The model under review builds one solid part; all positions refer to its coordinate system, in mm. A direction names the side the tool comes from. Coordinates: 2 decimals unless noted, no trailing zeros. Loops run counter-clockwise (first coordinate to the right, second up) from the corner with the lowest first, then second, coordinate; pieces in that order, holes last. Notation, with made-up numbers: M 74.5,-39.75 L 83.5,-39.75 A16 ccw 83.5,-30.75 Z; hole C -17,23.5 d10. An arc over 180 degrees is marked long. Return JSON: item names as keys, results as strings.
Autodesk Fusion 360 part; units mm, degrees
sketch "Sketch1" plane through (0, 0, 0) normal (0, 0, 1) x (1, 0, 0)
  line L0 (5, 5) -> (130, 5)
  line L1 (130, 5) -> (130, 205)
  line L2 (130, 205) -> (5, 205)
  line L3 (5, 205) -> (5, 5)
  line L4 (5, 5) -> (31.5, 5)
  line L5 (31.5, 5) -> (31.5, 45)
  line L6 (31.5, 45) -> (103.5, 45)
  line L7 (103.5, 45) -> (103.5, 184)
  line L8 (103.5, 184) -> (31.5, 184)
  line L9 (31.5, 184) -> (31.5, 45)
  line L10 (31.5, 45) -> (36.5, 45)
  line L11 (36.5, 45) -> (36.5, 50)
  circle A0 centre (36.5, 50) radius 1.75
  line L12 (103.5, 45) -> (98.5, 45)
  line L13 (98.5, 45) -> (98.5, 50)
  circle A1 centre (98.5, 50) radius 1.75
  line L14 (31.5, 184) -> (36.5, 184)
  line L15 (36.5, 184) -> (36.5, 179)
  circle A2 centre (36.5, 179) radius 1.75
  line L16 (103.5, 184) -> (103.5, 179)
  line L17 (103.5, 179) -> (98.5, 179)
  circle A3 centre (98.5, 179) radius 1.75
  dimension "d1" = 125
  dimension "d2" = 200
  dimension "d58" = 26.5
  dimension "d59" = 40
  dimension "d60" = 72
  dimension "d61" = 139
  dimension "d62" = 5
  dimension "d63" = 5
  dimension "d64" = 3.5
  dimension "d65" = 5
  dimension "d66" = 5
  dimension "d67" = 3.5
  dimension "d68" = 5
  dimension "d69" = 5
  dimension "d70" = 3.5
  dimension "d71" = 5
  dimension "d72" = 5
  dimension "d73" = 3.5
extrude "Extrude1" add sketch "Sketch1" along normal blind 3 contours L6 L7 L8 L9 L10 L12 L14 L16 | L0 L1 L2 L3 L4
sketch "Sketch2" plane through (0, 0, 0) normal (0, 0, -1) x (-1, 0, 0)
  line L0 (-5, 5) -> (-5, 205)
  line L1 (-5, 205) -> (-130, 205)
  line L2 (-130, 205) -> (-130, 5)
  line L3 (-130, 5) -> (-5, 5)
  line L4 (-130, 205) -> (-130, 185)
  line L5 (-130, 5) -> (-130, 25)
  line L6 (-130, 185) -> (-127, 185)
  line L7 (-127, 185) -> (-127, 25)
  line L8 (-127, 25) -> (-130, 25)
  line L9 (-130, 25) -> (-130, 185)
  line L10 (-8, 185) -> (-8, 25)
  line L11 (-5, 25) -> (-5, 185)
  line L12 (-5, 185) -> (-8, 185)
  line L13 (-5, 205) -> (-5, 185)
  line L14 (-8, 25) -> (-5, 25)
  line L15 (-5, 5) -> (-5, 25)
  line L16 (-5, 205) -> (-10.3033, 199.6967)
  line L17 (-5, 205) -> (-10, 205) construction
  line L18 (-5, 5) -> (-10.3033, 10.3033)
  line L19 (-5, 5) -> (-10, 5) construction
  circle A0 centre (-10.3033, 10.3033) radius 2.5
  circle A1 centre (-10.3033, 199.6967) radius 2.5
  circle A2 centre (-124.6967, 199.6967) radius 2.5
  line L20 (-130, 205) -> (-124.6967, 199.6967)
  line L21 (-130, 5) -> (-124.6967, 10.3033)
  circle A3 centre (-124.6967, 10.3033) radius 2.5
  line L22 (-67.5, 205) -> (-130, 205)
  line L23 (-67.5, 205) -> (-5, 205)
  line L24 (-30, 205) -> (-30, 5)
  line L25 (-30, 205) -> (-5, 205)
  line L26 (-5, 185) -> (-5, 205)
  line L27 (-5, 185) -> (-8, 185)
  line L28 (-8, 185) -> (-8, 25)
  line L29 (-8, 25) -> (-5, 25)
  line L30 (-5, 25) -> (-5, 5)
  line L31 (-5, 5) -> (-30, 5)
  line L32 (-30, 205) -> (-67.5, 205)
  line L33 (-67.5, 5) -> (-36.25, 5)
  line L34 (-67.5, 5) -> (-98.75, 5)
  line L35 (-67.5, 205) -> (-130, 205)
  line L36 (-130, 205) -> (-130, 185)
  line L37 (-127, 185) -> (-127, 25)
  line L38 (-130, 5) -> (-130, 25)
  line L39 (-130, 5) -> (-98.75, 5)
  line L40 (-130, 185) -> (-127, 185)
  line L41 (-30, 205) -> (-55, 205)
  line L42 (-55, 205) -> (-55, 5)
  line L43 (-55, 5) -> (-30, 5)
  line L44 (-30, 5) -> (-30, 205)
  line L45 (-55, 205) -> (-80, 205)
  line L46 (-80, 205) -> (-80, 5)
  line L47 (-80, 5) -> (-55, 5)
  line L48 (-55, 5) -> (-55, 205)
  line L49 (-80, 205) -> (-105, 205)
  line L50 (-105, 205) -> (-105, 5)
  line L51 (-105, 5) -> (-80, 5)
  line L52 (-80, 5) -> (-80, 205)
  circle A4 centre (-98.5, 50) radius 1.75
  circle A5 centre (-98.5, 179) radius 1.75
  circle A6 centre (-36.5, 50) radius 1.75
  circle A7 centre (-36.5, 179) radius 1.75
  dimension "d6" = 20
  dimension "d7" = 3
  dimension "d8" = 45
  dimension "d9" = 7.5
  dimension "d10" = 45
  dimension "d11" = 7.5
  dimension "d12" = 5
  dimension "d13" = 5
  dimension "d20" = 160
  dimension "d21" = 20
  dimension "d23" = 200
  dimension "d38" = 25
  dimension "d39" = 25
  dimension "d40" = 25
  dimension "d41" = 25
extrude "Extrude2" cut sketch "Sketch2" against normal blind 3 contours A1
extrude "Extrude3" cut sketch "Sketch2" against normal blind 3 contours A0 | A2 | A3
extrude "Extrude4" add sketch "Sketch2" along normal blind 5 contours L0 L10 L11 L12 L14 L27 L28 L29 | L2 L6 L7 L8 L9 L37 L40
sketch "Sketch3" plane through (0, 0, 3) normal (0, 0, 1) x (1, 0, 0)
  circle A0 centre (124.6967, 199.6967) radius 2.5
  circle A1 centre (124.6967, 10.3033) radius 2.5
  circle A2 centre (10.3033, 10.3033) radius 2.5
  circle A3 centre (10.3033, 199.6967) radius 2.5
  line L0 (5, 205) -> (5, 5)
  line L1 (5, 5) -> (130, 5)
  line L2 (130, 5) -> (130, 205)
  line L3 (130, 205) -> (5, 205)
  line L4 (5, 5) -> (5, 35)
  line L5 (5, 5) -> (30, 5)
  line L6 (5, 35) -> (17.5, 35)
  circle A4 centre (17.5, 35) radius 4.5
  line L7 (17.5, 35) -> (17.5, 67.5)
  circle A5 centre (17.5, 67.5) radius 4.5
  line L8 (17.5, 67.5) -> (17.5, 120)
  circle A6 centre (17.5, 120) radius 3.5
  line L9 (17.5, 120) -> (17.5, 140)
  circle A7 centre (17.5, 140) radius 3.5
  line L10 (17.5, 140) -> (17.5, 160)
  circle A8 centre (17.5, 160) radius 3.5
  line L11 (130, 5) -> (98.75, 5)
  line L12 (30, 5) -> (30, 205)
  circle A9 centre (42.5, 160) radius 3.5
  circle A10 centre (42.5, 140) radius 3.5
  circle A11 centre (42.5, 67.5) radius 4.5
  circle A12 centre (42.5, 120) radius 3.5
  circle A13 centre (42.5, 35) radius 4.5
  line L13 (55, 205) -> (55, 5)
  circle A14 centre (67.5, 160) radius 3.5
  circle A15 centre (67.5, 140) radius 3.5
  circle A16 centre (67.5, 67.5) radius 4.5
  circle A17 centre (67.5, 35) radius 4.5
  line L14 (80, 5) -> (80, 205)
  circle A18 centre (92.5, 160) radius 3.5
  circle A19 centre (92.5, 67.5) radius 4.5
  circle A20 centre (92.5, 35) radius 4.5
  line L15 (80, 205) -> (80, 5)
  circle A21 centre (117.5, 160) radius 3.5
  circle A22 centre (117.5, 140) radius 3.5
  circle A23 centre (117.5, 120) radius 3.5
  circle A24 centre (117.5, 67.5) radius 4.5
  circle A25 centre (117.5, 35) radius 4.5
  line L16 (17.5, 67.5) -> (17.5, 82.5)
  circle A26 centre (17.5, 82.5) radius 2.5
  circle A27 centre (42.5, 82.5) radius 2.5
  circle A28 centre (67.5, 82.5) radius 2.5
  circle A29 centre (92.5, 82.5) radius 2.5
  line L17 (105, 205) -> (105, 5)
  circle A30 centre (117.5, 82.5) radius 2.5
  circle A31 centre (98.5, 50) radius 1.75
  circle A32 centre (98.5, 179) radius 1.75
  circle A33 centre (36.5, 50) radius 1.75
  circle A34 centre (36.5, 179) radius 1.75
  dimension "d24" = 30
  dimension "d25" = 31.25
  dimension "d26" = 12.5
  dimension "d27" = 9
  dimension "d28" = 32.5
  dimension "d29" = 9
  dimension "d30" = 52.5
  dimension "d31" = 7
  dimension "d32" = 20
  dimension "d33" = 7
  dimension "d34" = 20
  dimension "d35" = 7
  dimension "d36" = 31.25
  dimension "d42" = 15
  dimension "d43" = 5
extrude "Extrude5" cut sketch "Sketch3" against normal blind 3 contours A8 | L9 A7 L10 | L9 A7 L10 | L8 A6 L9 | L8 A6 L9 | L8 L16 A26 | L8 L16 A26 | L7 A5 L8 L16 | L7 A5 L8 L16 | L6 A4 L7 | L6 A4 L7 | A9 | A10 | A11 | A12 | A13 | A14 | A15 | A16 | A17 | A18 | A19 | A20 | A21 | A22 | A23 | A24 | A25 | A27 | A28 | A29 | A30
sketch "Sketch4" plane through (0, 0, 3) normal (0, 0, 1) x (1, 0, 0)
  circle A0 centre (117.5, 82.5) radius 2.5
  circle A1 centre (42.5, 160) radius 3.5
  circle A2 centre (92.5, 67.5) radius 4.5
  circle A3 centre (67.5, 82.5) radius 2.5
  circle A4 centre (42.5, 82.5) radius 2.5
  circle A5 centre (17.5, 67.5) radius 4.5
  circle A6 centre (17.5, 160) radius 3.5
  circle A7 centre (17.5, 82.5) radius 2.5
  circle A8 centre (42.5, 67.5) radius 4.5
  circle A9 centre (67.5, 140) radius 3.5
  circle A10 centre (92.5, 35) radius 4.5
  circle A11 centre (67.5, 160) radius 3.5
  circle A12 centre (117.5, 120) radius 3.5
  circle A13 centre (117.5, 67.5) radius 4.5
  circle A14 centre (117.5, 160) radius 3.5
  circle A15 centre (92.5, 82.5) radius 2.5
  circle A16 centre (67.5, 67.5) radius 4.5
  circle A17 centre (42.5, 120) radius 3.5
  circle A18 centre (17.5, 35) radius 4.5
  circle A19 centre (17.5, 140) radius 3.5
  circle A20 centre (17.5, 120) radius 3.5
  circle A21 centre (42.5, 35) radius 4.5
  circle A22 centre (42.5, 140) radius 3.5
  circle A23 centre (67.5, 35) radius 4.5
  circle A24 centre (92.5, 160) radius 3.5
  circle A25 centre (117.5, 140) radius 3.5
  circle A26 centre (117.5, 35) radius 4.5
  circle A27 centre (124.6967, 199.6967) radius 2.5
  circle A28 centre (124.6967, 10.3033) radius 2.5
  circle A29 centre (10.3033, 10.3033) radius 2.5
  circle A30 centre (10.3033, 199.6967) radius 2.5
  line L0 (5, 205) -> (5, 5)
  line L1 (5, 5) -> (130, 5)
  line L2 (130, 5) -> (130, 205)
  line L3 (130, 205) -> (5, 205)
  line L4 (5, 205) -> (17.5, 205)
  line L5 (17.5, 205) -> (17.5, 5)
  line L6 (17.5, 205) -> (42.5, 205)
  line L7 (42.5, 205) -> (42.5, 5)
  line L8 (42.5, 5) -> (17.5, 5)
  line L9 (17.5, 5) -> (17.5, 205)
  line L10 (42.5, 205) -> (67.5, 205)
  line L11 (67.5, 205) -> (67.5, 5)
  line L12 (67.5, 5) -> (42.5, 5)
  line L13 (42.5, 5) -> (42.5, 205)
  line L14 (67.5, 205) -> (92.5, 205)
  line L15 (92.5, 205) -> (92.5, 5)
  line L16 (92.5, 5) -> (67.5, 5)
  line L17 (67.5, 5) -> (67.5, 205)
  line L18 (92.5, 205) -> (117.5, 205)
  line L19 (117.5, 205) -> (117.5, 5)
  line L20 (117.5, 5) -> (92.5, 5)
  line L21 (92.5, 5) -> (92.5, 205)
  line L22 (5, 205) -> (5, 185)
  line L23 (5, 185) -> (130, 185)
  circle A31 centre (98.5, 50) radius 1.75
  circle A32 centre (98.5, 179) radius 1.75
  circle A33 centre (36.5, 50) radius 1.75
  circle A34 centre (36.5, 179) radius 1.75
  dimension "d47" = 12.5
  dimension "d49" = 25
  dimension "d50" = 200
  dimension "d51" = 25
  dimension "d52" = 25
  dimension "d53" = 200
  dimension "d54" = 25
  dimension "d56" = 20
  dimension "d57" = 125
sketch "Sketch5" plane through (0, 0, 3) normal (0, 0, 1) x (1, 0, 0)
chamfer "Chamfer1" distance 5 angle 45 4 edges at (6.5, 185, -5) (6.5, 25, -5) (128.5, 25, -5) (128.5, 185, -5)
sketch "Sketch6" plane through (0, 0, 0) normal (0, 0, 1) x (1, 0, 0)
  circle A0 centre (98.5, 179) radius 3.5
  circle A1 centre (98.5, 50) radius 3.5
  circle A2 centre (98.5, 50) radius 1.75
  circle A3 centre (98.5, 179) radius 1.75
  line L0 (67.5, 205) -> (67.5, 5)
  circle A4 centre (36.5, 179) radius 3.5
  circle A5 centre (36.5, 179) radius 1.75
  circle A6 centre (36.5, 50) radius 3.5
  circle A7 centre (36.5, 50) radius 1.75
  dimension "d75" = 7
  dimension "d76" = 7
  dimension "d77" = 3.5
  dimension "d78" = 3.5
extrude "Extrude6" add sketch "Sketch6" against normal blind 20
1. Add section A-A on y = 35. Give the boundary of the cut face in (x, z).
Check values:
{"outline": "M 5,-5 L 8,-5 L 8,0 L 13,0 L 13,3 L 5,3 Z; M 22,0 L 38,0 L 38,3 L 22,3 Z; M 47,0 L 63,0 L 63,3 L 47,3 Z; M 72,0 L 88,0 L 88,3 L 72,3 Z; M 97,0 L 113,0 L 113,3 L 97,3 Z; M 122,0 L 127,0 L 127,-5 L 130,-5 L 130,3 L 122,3 Z"}
2. To check wall thickness, follow line 1 (Y direction, x = 98.5, z = -14.5); line 2 (X direction, y = 170.5, z = -4.25); line 3 (Z direction, x = 24, y = 122). State the ranges of each line that lie inside material, in increasing order.
Check values:
{"line 1": "46.5 to 48.25, 51.75 to 53.5, 175.5 to 177.25, 180.75 to 182.5", "line 2": "5 to 8, 127 to 130", "line 3": "0 to 3"}
3. The part is to be moulded in two halves that separate along X. For faces 1 (the face through (5, 106, -1)), 2 (the face through (68.84, 84.61, 1.52)), 3 (the face through (99, 181, -20)), 4 (the face through (44.919, 71.294, 1.521)), say which applies: released by +X, released by -X, zero draft, split by the parting line, or undercut.
Check values:
{"face 1": "released by -X", "face 2": "undercut", "face 3": "zero draft", "face 4": "undercut"}
4. Add section D-D on y = 120. Give the boundary of the cut face in (x, z), plus the area to 3 significant figures.
Check values:
{"outline": "M 5,-5 L 8,-5 L 8,0 L 14,0 L 14,3 L 5,3 Z; M 21,0 L 39,0 L 39,3 L 21,3 Z; M 46,0 L 114,0 L 114,3 L 46,3 Z; M 121,0 L 127,0 L 127,-5 L 130,-5 L 130,3 L 121,3 Z", "area": "342 mm²"}
5. Add section C-C on x = 17.5. Give the boundary of the cut face in (y, z), plus the area to 3 significant figures.
Check values:
{"outline": "M 5,0 L 30.5,0 L 30.5,3 L 5,3 Z; M 39.5,0 L 63,0 L 63,3 L 39.5,3 Z; M 72,0 L 80,0 L 80,3 L 72,3 Z; M 85,0 L 116.5,0 L 116.5,3 L 85,3 Z; M 123.5,0 L 136.5,0 L 136.5,3 L 123.5,3 Z; M 143.5,0 L 156.5,0 L 156.5,3 L 143.5,3 Z; M 163.5,0 L 205,0 L 205,3 L 163.5,3 Z", "area": "468 mm²"}
6. Machinability: for faces 5 (the face through (8, 106, -2)), 6 (the face through (7, 182, -3)), 7 (the face through (33.7, 176.9, -9.9)), which of the approach directions +Z, -Z, +X, -X, +Y, -Y give a long, thin tool a straight path to every point of the face, cutting with its end or side? Answer none if there is none.
Check values:
{"face 5": "-Z, +Y, -Y", "face 6": "-Z, -X, +Y", "face 7": "-Z"}
7. Insertion check: pin 1 Ø10.5 at (x, y) = (42.5, 67.5) entering from -Z; pin 2 Ø0.9 at (x, y) = (128, 110.5) entering from -Z. Each pin has a flat end and moves straight along its axis. Give the tip position at first contact, or say it passes through.
Check values:
{"pin 1": "z = 0", "pin 2": "z = -5"}
8. Add section B-B on z = -15.75. Give the boundary of the cut face in (x, y).
Check values:
{"outline": "C 36.5,50 d7; C 36.5,179 d7; C 98.5,50 d7; C 98.5,179 d7; hole C 36.5,50 d3.5; hole C 36.5,179 d3.5; hole C 98.5,50 d3.5; hole C 98.5,179 d3.5"}
